Geometry: see drawing. Coordinates: mm, zero at the bounding-box minimum. A direction names the side the tool comes from. Give positions to 0.01 mm unless a question says otherwise; leave off trailing zeros. Write each loop counter-clockwise with the first axis right and the second up, starting at its lowest first coordinate (ties: lowest second). Pieces come first, ordered by that corner, then holes. Notation, with made-up numbers: (-36, 15.25) -> (-7, 15.25) arc R19 cw to (-7, 25.25) -> close; hole circle Ø9 at (-37, 35). An arc over 180 degrees is marked (long way). Answer as a JSON object with one key per item and string values. Group by question number.
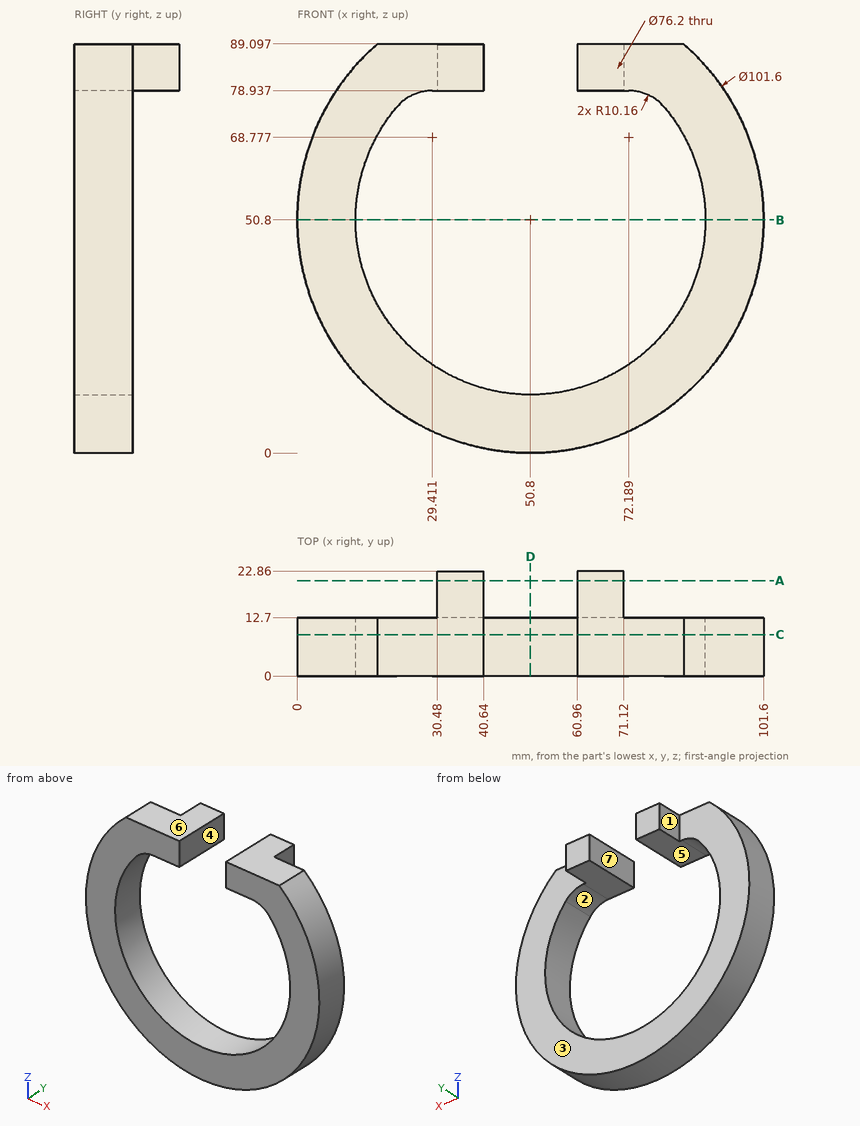
1. Contact query for flat-ended pins moving along their axis: pin 1 Ø3.5 at (x, y) = (37, 10) entering from -Z; pin 2 Ø10 at (y, z) = (6.5, 48.5) entering from -X; pin 3 Ø3 at (y, z) = (17, 82) entering from -X. Output: stop coordinate, or through.
2. Reachability of the marked faces 5, 6 and 7 from +Z, -Z, +X, -X, +Y, -Y: full face, straight path, thin tool, end or side. Return the list, or none.
3. Line query: line 1 (X direction, y = 11, z = 50.5); line 2 (Z direction, x = 27.5, y = 10.75) (1 decimal); line 3 (Z direction, x = 72, y = 4.5) (1 decimal). Output: solid intervals per line, ascending.
4. Section A-A (y = 20.75). Return the cut outline in (x, z), plus the area to 3 significant figures.
5. Section C-C (y = 9). Return the cut outline in (x, z).
6. Mould query, pull axis X, two halves, no side actions, for the marked faces 1, 2, 3 and 4. Classes: pulls with the +X half, pulls with the -X half, needs draft (parallel to the pull), parting line crosses it, or undercut.
7. Section B-B (z = 50.8). Return the cut outline in (x, y), plus the area to 3 significant figures.
8. Section D-D (x = 50.8). Return the cut outline in (y, z), plus the area to 3 significant figures.
Working result:
{
 "1": {"pin 1": "stops at z = 1.45", "pin 2": "stops at x = 0", "pin 3": "stops at x = 30.48"},
 "2": {"face 5": "+Y, -Y", "face 6": "+Z, +X, -X, +Y, -Y", "face 7": "+Z, +Y, -Y"},
 "3": {"line 1": "x = 0 to 12.7, 88.9 to 101.6", "line 2": "z = 5.7 to 20.7, 78.8 to 89.1", "line 3": "z = 4.6 to 19.1, 78.9 to 89.1"},
 "4": {"outline": "(30.48, 78.94) -> (40.64, 78.94) -> (40.64, 89.1) -> (30.48, 89.1) -> close; (60.96, 78.94) -> (71.12, 78.94) -> (71.12, 89.1) -> (60.96, 89.1) -> close", "area": "206 mm^2"},
 "5": {"outline": "(17.42, 89.1) arc R50.8 ccw (long way) to (84.18, 89.1) -> (60.96, 89.1) -> (60.96, 78.94) -> (72.19, 78.94) arc R10.16 cw to (79.97, 75.31) arc R38.1 cw (long way) to (21.63, 75.31) arc R10.16 cw to (29.41, 78.94) -> (40.64, 78.94) -> (40.64, 89.1) -> close"},
 "6": {"face 1": "pulls with the -X half", "face 2": "undercut", "face 3": "needs draft", "face 4": "undercut"},
 "7": {"outline": "(0, 0) -> (12.7, 0) -> (12.7, 12.7) -> (0, 12.7) -> close; (88.9, 0) -> (101.6, 0) -> (101.6, 12.7) -> (88.9, 12.7) -> close", "area": "323 mm^2"},
 "8": {"outline": "(0, 0) -> (12.7, 0) -> (12.7, 12.7) -> (0, 12.7) -> close", "area": "161 mm^2"}
}
